The model under review builds one solid part; all positions refer to its coordinate system, in mm. A direction names the side the tool comes from. Give positions to 0.01 mm unless a question says otherwise; leave off trailing zeros. Write each loop counter-clockwise with the first axis right and the second up, starting at its lowest first coordinate (ties: lowest second). Pieces come first, ordered by that corner, then holes. Notation, with made-up numbers: (34, 31) - (86, 31) arc R21 cw to (86, 38) - close; hole circle Ø10 at (68.25, 63.5). An arc over 180 degrees is marked (long way). One line per question, with ' | ' between items. Start each with the question number.
```python
from build123d import *

# Parameters (mm, degrees)
F0_W     = 76.2
F0_H     = 101.6
F1_DEPTH = 12.7
F2_W     = 12.7
F2_H     = 101.6
F3_DEPTH = 50.8
F4_W     = 12.7
F4_H     = 50.8
F5_DEPTH = 50.8
F6_R     = 12.7
F7_DEPTH = 25.4


with BuildPart() as f1:
    # F0 (on Front) → F1 (new body)
    with BuildSketch(Plane.XZ):
        Rectangle(F0_W, F0_H)
    extrude(amount=F1_DEPTH)

    # F2 (on face) → F3 (join)
    with BuildSketch(Plane.XZ.offset(12.7)):
        Rectangle(F2_W, F2_H)
    extrude(amount=F3_DEPTH)

    # F4 (on face) → F5 (join)
    with BuildSketch(Plane.XY.offset(50.8)):
        with Locations((0, -38.1)):
            Rectangle(F4_W, F4_H)
    extrude(amount=F5_DEPTH)

    # F6 (on face) → F7 (cut)
    with BuildSketch(Plane.YZ.offset(6.35)):
        with Locations((-38.1, 82.55)):
            Circle(F6_R)
        with BuildLine():
            ThreePointArc((-12.7, -50.8), (-48.635426, 11.861504), (-63.5, 82.55))
            Line((-63.5, 82.55), (-133.589551, -36.487788))
            Line((-133.589551, -36.487788), (-38.791277, -66.6712))
            Line((-38.791277, -66.6712), (-12.7, -50.8))
        make_face()
        with BuildLine():
            ThreePointArc((-63.5, 82.55), (-38.1, 101.6), (-12.7, 82.55))
            Line((-12.7, 82.55), (0, 103.250235))
            Line((0, 103.250235), (-76.800019, 103.250235))
            Line((-76.800019, 103.250235), (-63.5, 82.55))
        make_face()
    extrude(amount=-F7_DEPTH, mode=Mode.SUBTRACT)


solid = f1.part
```
Item 1: Machinability: for faces 1 (the cylindrical face through (0.089, -38.577, 101.596)), 2 (the flat face through (38.1, -6, -1)), 3 (the flat face through (0, -12.7, 66)), 4 (the flat face through (-22, -12.7, 1)), 5 (the flat face through (6.35, -33, 41)), which of the approach directions +Z, -Z, +X, -X, +Y, -Y give a long, thin tool a straight path to every point of the face, cutting with its end or side? Answer none if there is none.
Item 2: Take a section at B-B (y = -31). Give the boundary of the cut face in (x, z).
Item 3: Clearance check with flat-ended pins moving along their axes: P1, Ø15, axis at y = -47, z = 16.5, coming from the -X side; P2, Ø8, axis at x = 7.5, y = -45.5, coming from the -Z side; P3, Ø5, axis at x = 7, z = -5.5, coming from the -Y side; P4, Ø5, axis at x = 10.5, z = 71.5, coming from the -Y side. State where each tip first meets the part, or that it passes through.
Item 4: Take a section at D-D (y = -9). Give the boundary of the cut face in (x, z), plus the area to 3 significant figures.
Item 5: Take a section at C-C (z = 79.5). Give the boundary of the cut face in (x, y).
Item 6: The part is to be moulded in two halves that separate along Y. For faces 6 (the flat face through (-1, 0, 1)), 7 (the cylindrical face through (0.09, -48.27, 10.91)), 8 (the flat face through (-1, -6, 50.8)), 9 (the cylindrical face through (0.089, -50.788, 83.108)), say which applies: +Y half, -Y half, draft (parallel to the pull), parting line (faces both ways), or undercut.
Item 7: Take a section at A-A (x = 1). Give the boundary of the cut face in (y, z), plus the area to 3 significant figures.
Item 8: For probe 1 along Y at (x, z) = (3, 82); probe 2 along X at (y, z) = (-13, -1); probe 3 along Y at (x, z) = (30, 36), list the stretches that pass through material, from the lowest coordinate up.
Check sheet entries:
1) face 1: +Z, +X, -X | face 2: +Z, -Z, +X, +Y, -Y | face 3: +Z, +X, -X, +Y | face 4: +Z, -Z, -X, -Y | face 5: +Z, -Z, +X, -Y
2) outline: (-6.35, -24.51) - (6.35, -24.51) - (6.35, 72.02) - (-6.35, 72.02) - close; (-6.35, 93.08) - (6.35, 93.08) - (6.35, 100.63) - (-6.35, 100.63) - close
3) P1: stops at x = -6.35 | P2: stops at z = -4.51 | P3: stops at y = -42.33 | P4: passes through
4) outline: (-38.1, -50.8) - (38.1, -50.8) - (38.1, 50.8) - (-38.1, 50.8) - close | area: 7,740 mm^2
5) outline: (-6.35, -63.33) - (6.35, -63.33) - (6.35, -50.43) - (-6.35, -50.43) - close; (-6.35, -25.77) - (6.35, -25.77) - (6.35, -12.7) - (-6.35, -12.7) - close
6) face 6: +Y half | face 7: -Y half | face 8: draft | face 9: undercut
7) outline: (-63.5, 82.55) arc R231.41 ccw to (-12.7, -50.8) - (0, -50.8) - (0, 50.8) - (-12.7, 50.8) - (-12.7, 82.55) arc R26.46 ccw to start; hole circle Ø25.4 at (-38.1, 82.55) | area: 5,960 mm^2
8) probe 1: y = -63.47 to -50.79, -25.41 to -12.7 | probe 2: x = -6.35 to 6.35 | probe 3: y = -12.7 to 0
